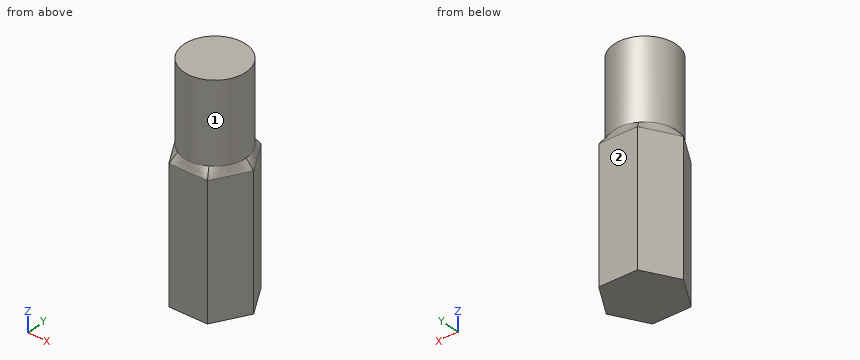
```python
from build123d import *

# Parameters (mm, degrees)
F1_DEPTH = 15
F3_R     = 3.5
F5_DEPTH = 9


with BuildPart() as f1:
    # F0 (on Top) → F1 (new body)
    with BuildSketch(Plane.XY):
        Polygon((2.1650635095, 3.75), (-2.1650635095, 3.75), (-4.3301270189, 0), (-2.1650635095, -3.75), (2.1650635095, -3.75), (4.3301270189, 0), align=None)
    extrude(amount=F1_DEPTH)

    # F1_face (on face) → F4 section 0
    with BuildSketch(Plane.XY.offset(15)):
        Polygon((4.3301270189, 0), (2.1650635095, 3.75), (-2.1650635095, 3.75), (-4.3301270189, 0), (-2.1650635095, -3.75), (2.1650635095, -3.75), align=None)
    # F3 (on offset) → F4 section 1
    with BuildSketch(Plane.XY.offset(16)):
        Circle(F3_R)
    loft()

    # F5 (add): a face of the model
    f5_faces = [f1.faces().sort_by_distance(p)[0] for p in [
        (0, 0, 16),
    ]]
    extrude(f5_faces, amount=F5_DEPTH)


solid = f1.part
```
Verification items for the finished model (mm, model axes). Face numbers are marked on the shaded views. A direction names the side the tool comes from. Round coordinates to 2 decimals unless told otherwise and drop trailing zeros. Write each loop counter-clockwise with the first axis right and the second up, starting at its lowest first coordinate (ties: lowest second). Pieces come first, ordered by that corner, then holes. Notation, with made-up numbers: (-18.75, -10.75) - (18.25, -10.75) arc R10 ccw to (18.25, -4.75) - close; hole circle Ø5 at (18.25, -34). An arc over 180 degrees is marked (long way). Answer as a JSON object with one key per item and string values. Group by question number.
Q1. Section check A-A, the plane z = 13. Enter the section's corners in (x, y).
Q2. Tool access check on the marked faces 1 and 2. Record the directions out of +Z, -Z, +X, -X, +Y, -Y that give a thin tool (end or side, any length) a straight path to the whole face; none if there is none.
Q3. Thickness scan on line 1 (X direction, y = -2.25, z = 8.5); line 2 (Y direction, x = 0, z = 17.5); line 3 (X direction, y = 2.75, z = 23.75). Record the ranges inside material, lowest first.
Q4. Go/stop test with flat-tipped pins: pin 1 Ø4 at (y, z) = (2.5, 18.5) entering from +X; pin 2 Ø2 at (y, z) = (2, 20) entering from +X. Record where each tip stops, or that it passes through.
Q5. Section check B-B, the plane z = 19.75. Enter the section's corners in (x, y), plus the area to 3 significant figures.
Found:
{
 "1": {"outline": "(-4.33, 0) - (-2.17, -3.75) - (2.17, -3.75) - (4.33, 0) - (2.17, 3.75) - (-2.17, 3.75) - close"},
 "2": {"face 1": "+Z", "face 2": "+Z, -Z, +X, -X, +Y"},
 "3": {"line 1": "x = -3.03 to 3.03", "line 2": "y = -3.5 to 3.5", "line 3": "x = -2.17 to 2.17"},
 "4": {"pin 1": "stops at x = 3.46", "pin 2": "stops at x = 3.35"},
 "5": {"outline": "circle Ø7 at (0, 0)", "area": "38.5 mm^2"}
}
